Design review of the part built by this model. Coordinates are the model's own, in mm. Coordinates: 2 decimals unless noted, no trailing zeros. Write each loop counter-clockwise with the first axis right and the second up, starting at its lowest first coordinate (ties: lowest second). Pieces come first, ordered by that corner, then holes. Notation, with made-up numbers: M 4.5,41.25 L 50.5,41.25 A13 cw 50.5,52.25 Z; hole C -13.5,7 d7. An arc over 180 degrees is marked long. Write each question's results on one line, items separated by ' | '. Start each with the question number.
Autodesk Inventor part; units mm, degrees
ref_plane "Work Plane1" through (25.4, 0, -89.027) normal (0, 0, -1) x (-1, 0, 0)
ref_plane "YZ Plane" through (0, 0, 0) normal (1, 0, 0) x (0, 1, 0)
ref_plane "XZ Plane" through (0, 0, 0) normal (0, 1, 0) x (-1, 0, 0)
sketch "Sketch1" plane through (0, 0, 0) normal (0, 1, 0) x (-1, 0, 0)
  line L0 (0, 0) -> (-25.4, 0)
  line L1 (-25.4, 0) -> (-25.4, -178.054)
  line L2 (-25.4, -178.054) -> (0, -178.054)
  line L3 (0, -178.054) -> (0, 0)
  dimension "d0" = 25.4
  dimension "d1" = 178.054
extrude "Extrusion1" add sketch "Sketch1" along normal blind 3.175
sketch "Sketch2" plane through (0, 3.175, 0) normal (0, 1, 0) x (1, 0, 0)
  line L0 (0, 178.054) -> (0, 0)
  line L1 (0, 0) -> (25.4, 0)
  point P0 (12.7, 17.78)
  dimension "d4" = 12.7
  dimension "d5" = 17.78
hole "Hole1" at (12.7, 3.175, -17.78) direction (0, -1, 0) diameter 6.35 end through all
ref_plane "Work Plane1" through (25.4, 0, -89.027) normal (0, 0, -1) x (-1, 0, 0)
mirror "Mirror1" about plane through (25.4, 0, -89.027) normal (0, 0, -1) of "Hole1"
sketch "Sketch3" plane through (25.4, 0, 0) normal (1, 0, 0) x (0, 0, -1)
  line L0 (0, 3.175) -> (178.054, 3.175)
  line L1 (0, 0) -> (178.054, 0)
  line L2 (0, 3.175) -> (178.054, 3.175)
  line L3 (178.054, 3.175) -> (178.054, 0)
  line L4 (178.054, 0) -> (0, 0)
  line L5 (0, 0) -> (0, 3.175)
extrude "Extrusion2" add sketch "Sketch3" along normal blind 12.7
sketch "Sketch4" plane through (0, 0, -178.054) normal (-1, 0, 0) x (0, 0, 1)
  line L0 (0, 0) -> (0, 3.175)
  line L1 (178.054, 0) -> (0, 0)
  line L2 (0, 0) -> (0, 3.175)
  line L3 (0, 3.175) -> (178.054, 3.175)
  line L4 (178.054, 3.175) -> (178.054, 0)
extrude "Extrusion3" add sketch "Sketch4" along normal blind 12.7
sketch "Sketch5" plane through (0, 3.175, 0) normal (0, 1, 0) x (1, 0, 0)
  line L0 (-12.7, 0) -> (-12.7, 178.054)
  line L1 (38.1, 0) -> (-12.7, 0)
  point P0 (0, 0)
  point P1 (12.7, 89.027)
  dimension "d17" = 25.4
  dimension "d18" = 89.027
hole "Hole2" at (12.7, 3.175, -89.027) direction (0, -1, 0) diameter 28.5496 end through all
sketch "Sketch6" plane through (0, 3.175, 0) normal (0, 1, 0) x (1, 0, 0)
  line L0 (38.1, 0) -> (-12.7, 0)
  line L1 (38.1, 0) -> (38.1, 178.054)
  point P0 (0, 0)
  point P1 (30.6578, 71.0692)
  dimension "d26" = 71.0692
  dimension "d27" = 7.4422
hole "Hole3" at (30.6578, 3.175, -71.0692) direction (0, -1, 0) diameter 4.0386 end through all
sketch "Sketch7" plane through (0, 3.175, 0) normal (0, 1, 0) x (1, 0, 0)
  line L0 (-12.7, 0) -> (-12.7, 178.054)
  line L1 (-12.7, 178.054) -> (38.1, 178.054)
  point P0 (0, 0)
  point P1 (-5.2578, 106.9848)
  dimension "d35" = 7.4422
  dimension "d36" = 71.0692
hole "Hole4" at (-5.2578, 3.175, -106.9848) direction (0, -1, 0) diameter 4.0386 end through all
properties part number "BAGMotor Beam"
Item 1: We need section C-C on y = 0.95. Count the separate pieces of the cut face and the enclosed holes in it, then the cut area to 3 significant figures.
Item 2: We need section A-A on x = 12.7. State the section outline as (y, z) points (3 decimals).
Item 3: Insertion check: pin 1 Ø8.5 at (x, z) = (12.7, -160.274) entering from -Y. The pin has a flat end and moves straight along its axis. Give the tip position at first contact, or say it passes through.
Item 4: We need section D-D on x = 3. State the section outline as (y, z) points (3 decimals).
Item 5: Wall thickness on L1, parallel to Z at x = 12.7, y = 1.6 (3 decimals); L2, parallel to X at y = 1.3, z = -17.78 (3 decimals); L3, parallel to Z at x = 3, y = 0.8: over which ranges is each line inside the solid? List them lowest first.
Item 6: Draft analysis for pull direction X (two halves, no side actions). For faces 1 (the cylindrical face through (14.63, 1.57, -20.3)), 2 (the flat face through (-12.7, 2, -90)), 3 (the flat face through (-4, 3.175, -90)), state which applies: released by +X, released by -X, zero draft, split by the parting line, or undercut.
Item 7: We need section B-B on z = -17.78. State the section outline as (x, y) points (3 decimals).
Answer:
1) separate pieces: 1 | enclosed holes: 5 | area: 8,320 mm^2
2) outline: M 0,-178.054 L 3.175,-178.054 L 3.175,-163.449 L 0,-163.449 Z; M 0,-157.099 L 3.175,-157.099 L 3.175,-103.302 L 0,-103.302 Z; M 0,-74.752 L 3.175,-74.752 L 3.175,-20.955 L 0,-20.955 Z; M 0,-14.605 L 3.175,-14.605 L 3.175,0 L 0,0 Z
3) pin 1: stops at y = 0
4) outline: M 0,-178.054 L 3.175,-178.054 L 3.175,-99.5 L 0,-99.5 Z; M 0,-78.554 L 3.175,-78.554 L 3.175,0 L 0,0 Z
5) L1: z = -178.054 to -163.449, -157.099 to -103.302, -74.752 to -20.955, -14.605 to 0 | L2: x = -12.7 to 9.525, 15.875 to 38.1 | L3: z = -178.05 to -99.5, -78.55 to 0
6) face 1: undercut | face 2: released by -X | face 3: zero draft
7) outline: M -12.7,0 L 9.525,0 L 9.525,3.175 L -12.7,3.175 Z; M 15.875,0 L 38.1,0 L 38.1,3.175 L 15.875,3.175 Z
